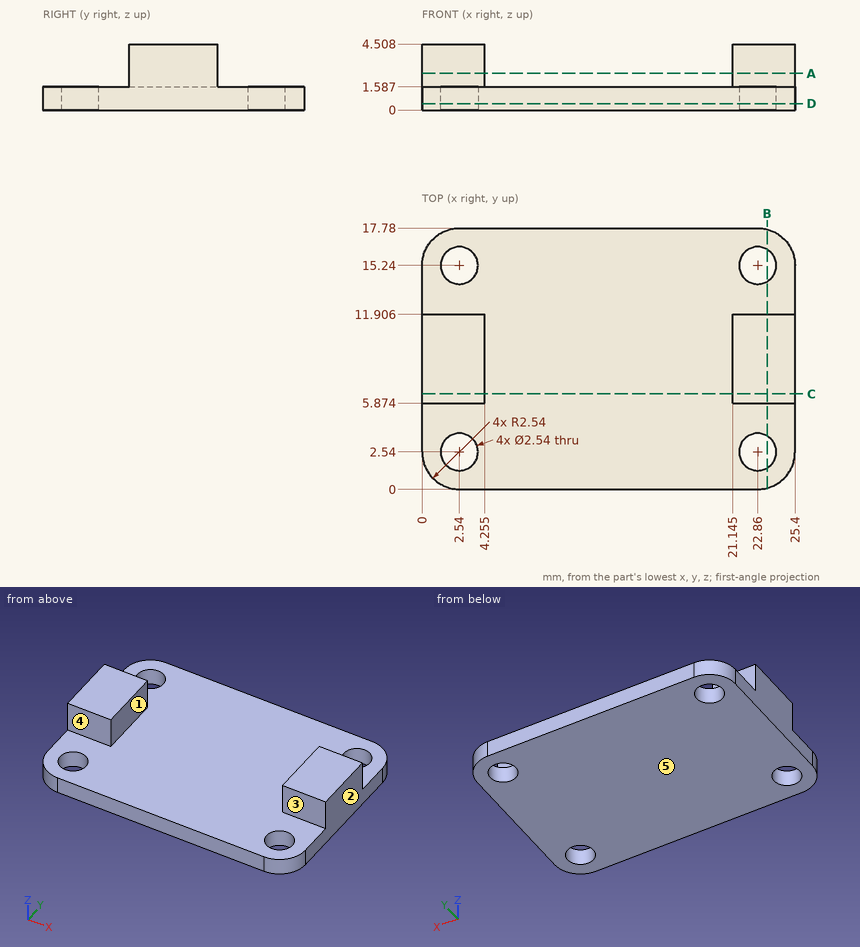
For this review, use the dimensioned drawing (mm, ordinates from the lowest corner) and the shaded views. A direction names the side the tool comes from. Give positions to 0.01 mm unless a question says otherwise; leave off trailing zeros. Order: outer loops, then holes, each group sorted by start corner. A loop starts at its lowest first (then second) coordinate and runs counter-clockwise, first axis right, second up. Notation, with made-up numbers: (85.25, 81.5) - (119.25, 81.5) arc R24 ccw to (119.25, 98.5) - close; hole circle Ø10 at (64.25, 74). An arc over 180 degrees is marked (long way). Use CSV: the item, a comma, the result in double quotes. Start each with the question number.
Q1. Clearance check with flat-ended pins moving along their axes: pin 1 Ø1.5 at (x, z) = (10.5, 3) entering from +Y; pin 2 Ø1.5 at (x, z) = (22.5, 3) entering from -Y. State where each tip first meets the part, or that it passes through.
Q2. To check wall thickness, follow line 1 along Y through (x, z) = (22.86, 0.5); line 2 along X through (y, z) = (9.75, 3) (1 decimal); line 3 along X through (y, z) = (15, 1.2). State the ranges of each line that lie inside material, in increasing order. Write a range as [from, to].
Q3. The part is to be moulded in two halves that separate along X. For the marked faces 1, 2 and 3, say which applies: +X half, -X half, draft (parallel to the pull), parting line (faces both ways), or undercut.
Q4. We need section B-B, the plane x = 23.5. Write out the cut boundary in (y, z).
Q5. We need section A-A, the plane z = 2.5. Write out the cut boundary in (x, y) (1 decimal).
Q6. Tool access review of the marked faces 4 and 5: name each direction out of +Z, -Z, +X, -X, +Y, -Y from which nothing blocks a thin tool from reaching the whole face with its end or side.
Q7. We need section C-C, the plane y = 6.5. Write out the cut boundary in (x, z) (1 decimal).
Q8. We need section D-D, the plane z = 0.45. Write out the cut boundary in (x, y), and give its area (3 significant figures).
Outcome:
1,pin 1,"passes through"
1,pin 2,"stops at y = 5.87"
2,line 1,"y = [0, 1.27], [3.81, 13.97], [16.51, 17.78]"
2,line 2,"x = [0, 4.3], [21.1, 25.4]"
2,line 3,"x = [0, 1.29], [3.79, 21.61], [24.11, 25.4]"
3,face 1,"undercut"
3,face 2,"+X half"
3,face 3,"draft"
4,outline,"(0.08, 0) - (1.44, 0) - (1.44, 1.59) - (0.08, 1.59) - close; (3.64, 0) - (14.14, 0) - (14.14, 1.59) - (11.91, 1.59) - (11.91, 4.51) - (5.87, 4.51) - (5.87, 1.59) - (3.64, 1.59) - close; (16.34, 0) - (17.7, 0) - (17.7, 1.59) - (16.34, 1.59) - close"
5,outline,"(0, 5.9) - (4.3, 5.9) - (4.3, 11.9) - (0, 11.9) - close; (21.1, 5.9) - (25.4, 5.9) - (25.4, 11.9) - (21.1, 11.9) - close"
6,face 4,"+Z, +X, -X, -Y"
6,face 5,"-Z, +X, -X, +Y, -Y"
7,outline,"(0, 0) - (25.4, 0) - (25.4, 4.5) - (21.1, 4.5) - (21.1, 1.6) - (4.3, 1.6) - (4.3, 4.5) - (0, 4.5) - close"
8,outline,"(0, 2.54) arc R2.54 ccw to (2.54, 0) - (22.86, 0) arc R2.54 ccw to (25.4, 2.54) - (25.4, 15.24) arc R2.54 ccw to (22.86, 17.78) - (2.54, 17.78) arc R2.54 ccw to (0, 15.24) - close; hole circle Ø2.54 at (2.54, 2.54); hole circle Ø2.54 at (2.54, 15.24); hole circle Ø2.54 at (22.86, 2.54); hole circle Ø2.54 at (22.86, 15.24)"
8,area,"426 mm^2"
